Geometry: see drawing. Coordinates: mm, zero at the bounding-box minimum. A direction names the side the tool comes from. Coordinates: 2 decimals unless noted, no trailing zeros. Write each loop counter-clockwise with the first axis right and the second up, starting at its lowest first coordinate (ties: lowest second). Pieces come first, ordered by that corner, then holes.
1) Set-up query: the marked faces 1 and 2. Return all of +Z, -Z, +X, -X, +Y, -Y with unobstructed straight access to the full face (end or side cutting, diameter ignored); none if empty.
2) Pin query (flat end, axial travel): pin 1 Ø2 at (x, y) = (2, 10.5) entering from +Z; pin 2 Ø0.6 at (x, y) = (18, 10.5) entering from +Z; pin 3 Ø4 at (x, z) = (5.5, 30) entering from -Y. Return the tip coordinate at first contact, or that it passes through.
3) Section query C-C (z = 17). Output: boundary loops of the cut face in (x, y).
4) Section query A-A (x = 10.25). Output: boundary loops of the cut face in (y, z).
5) Section query D-D (x = 2.25). Output: boundary loops of the cut face in (y, z), then the cut area to 3 significant figures.
6) Line query: L1, parallel to Y at x = 10.25, z = 33.2; L2, parallel to Y at x = 18.25, z = 33.1; L3, parallel to Z at x = 18.25, y = 15.25. Output: solid intervals per line, ascending.
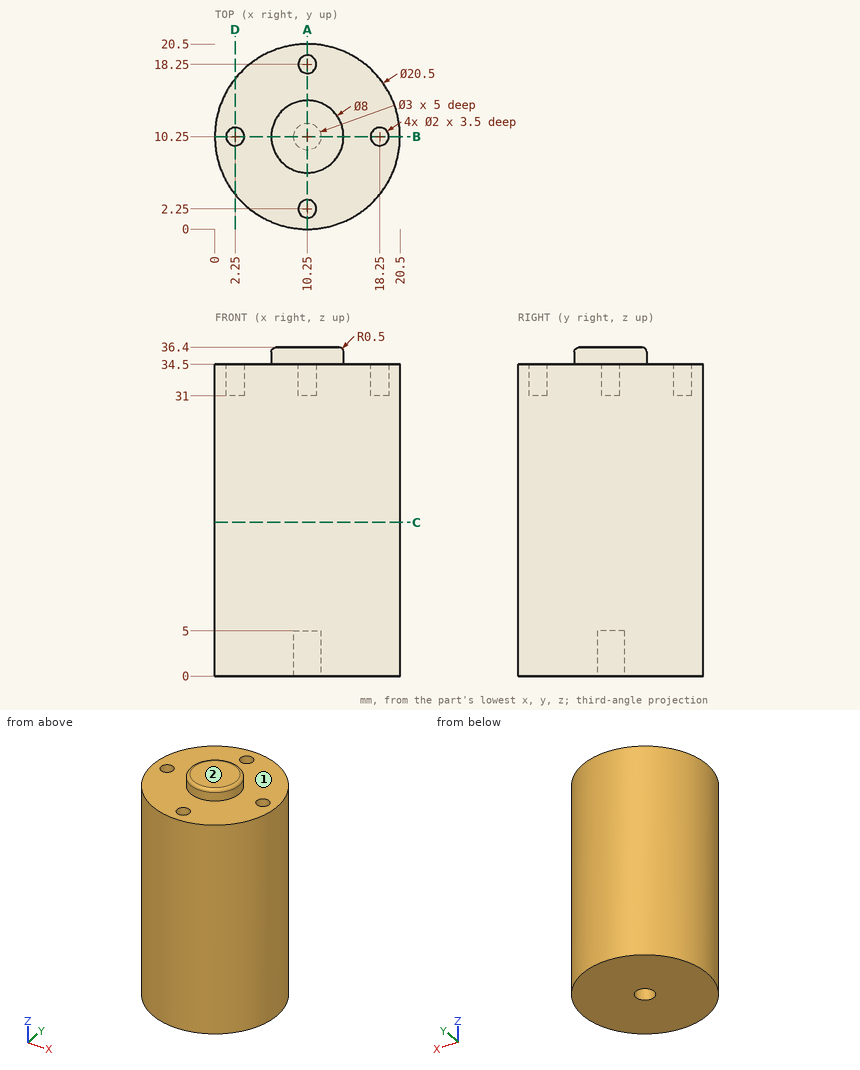
Answer:
1. face 1: +Z
1. face 2: +Z, +X, -X, +Y, -Y
2. pin 1: stops at z = 34.5
2. pin 2: stops at z = 31
2. pin 3: stops at y = 0.38
3. outline: circle Ø20.5 at (10.25, 10.25)
4. outline: (0, 0) - (8.75, 0) - (8.75, 5) - (11.75, 5) - (11.75, 0) - (20.5, 0) - (20.5, 34.5) - (19.25, 34.5) - (19.25, 31) - (17.25, 31) - (17.25, 34.5) - (14.25, 34.5) - (14.25, 35.9) arc R0.5 ccw to (13.75, 36.4) - (6.75, 36.4) arc R0.5 ccw to (6.25, 35.9) - (6.25, 34.5) - (3.25, 34.5) - (3.25, 31) - (1.25, 31) - (1.25, 34.5) - (0, 34.5) - close
5. outline: (3.84, 0) - (16.66, 0) - (16.66, 34.5) - (11.25, 34.5) - (11.25, 31) - (9.25, 31) - (9.25, 34.5) - (3.84, 34.5) - close
5. area: 435 mm2
6. L1: y = 0 to 1.25, 3.25 to 17.25, 19.25 to 20.5
6. L2: y = 3.84 to 9.25, 11.25 to 16.66
6. L3: z = 0 to 34.5
